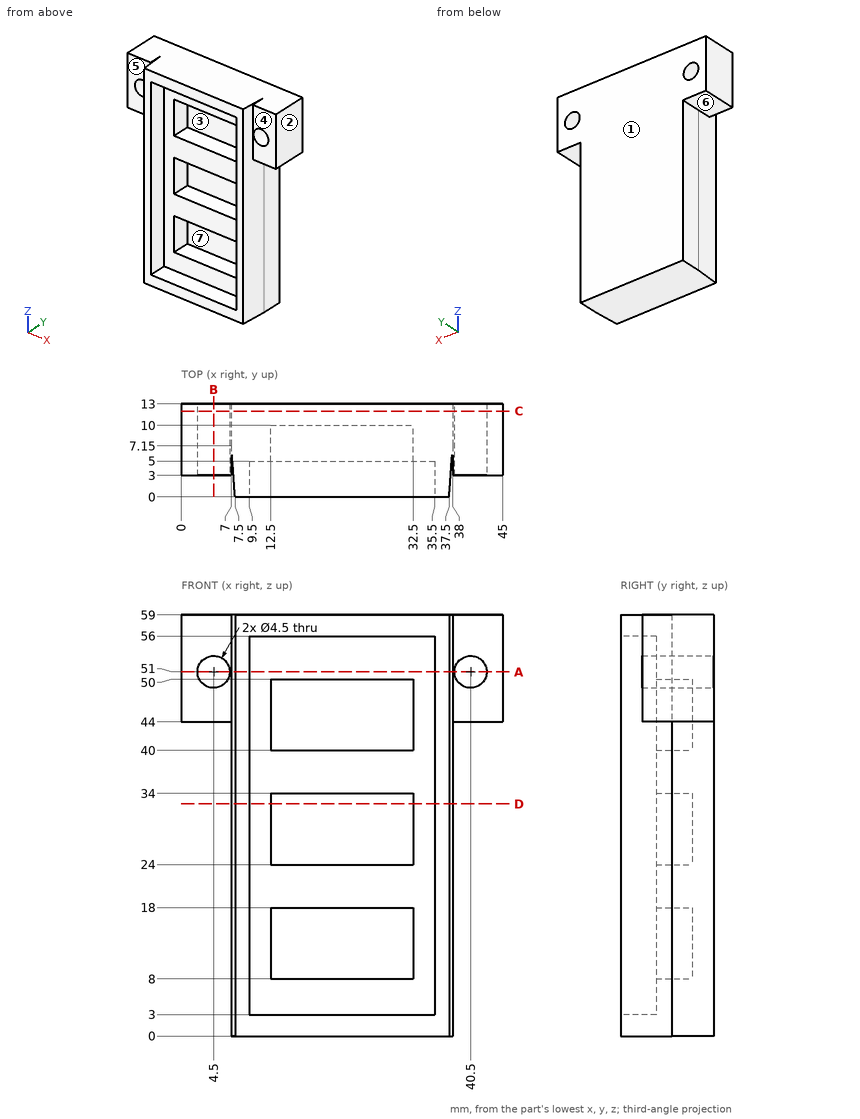
Print and shaded views of the part. All mm, measured from the part's lowest x, y and z. A direction names the side the tool comes from. Coordinates: 2 decimals unless noted, no trailing zeros. Loops run counter-clockwise (first coordinate to the right, second up) from the corner with the lowest first, then second, coordinate; pieces in that order, holes last. Notation, with made-up numbers: M 58.25,35.25 L 69.25,35.25 A12 cw 69.25,58.25 Z; hole C 86,33.5 d10. An arc over 180 degrees is marked long. Use a Markdown table: item, result. Add a question column.
Q1. Which spindle directions (+Z, -Z, +X, -X, +Y, -Y) get a long thin tool onto all of the face, cutting with end or side? Do the marked faces 4, 5, 6 and 7. Say none if no direction does.
Q2. Probe L1, parallel to Z at x = 18.5, y = 6; L2, parallel to X at y = 9.25, z = 51; L3, parallel to Z at x = 4.5, y = 10.75. List the from-to ranges inside material, lowest first.
Q3. Cut at B-B (x = 4.5). Write the cut outline in (y, z).
Q4. Mould opens along X. For the marked faces 1, 2 and 3 say: +X half, -X half, draft (parallel to the pull), parting line (faces both ways), or undercut.
Q5. Cut at D-D (z = 32.5). Write the cut outline in (x, y).
Q6. Cut at C-C (y = 12). Write the cut outline in (x, z), and give its area (3 significant figures).
Q7. Pin check, flat tips, straight feed: P1, Ø10, axis at x = 18.5, z = 25, coming from the -Y side; P2, Ø5, axis at x = 18.5, z = 28, coming from the -Y side; P3, Ø1.5, axis at y = 7.5, z = 12.5, coming from the +X side. Stop position of each tip, or through.
Q8. Cut at A-A (z = 51). Write the cut outline in (x, y).
Worked out:
| question | item | result |
|---|---|---|
| 1 | face 4 | +Z, -Z, +X, -Y |
| 1 | face 5 | +Z, -Z, -X, -Y |
| 1 | face 6 | -Z, -X, +Y, -Y |
| 1 | face 7 | -Y |
| 2 | L1 | z = 0 to 8, 18 to 24, 34 to 40, 50 to 59 |
| 2 | L2 | x = 0 to 2.25, 6.75 to 38.25, 42.75 to 45 |
| 2 | L3 | z = 44 to 48.75, 53.25 to 59 |
| 3 | outline | M 3,44 L 13,44 L 13,48.75 L 3,48.75 Z; M 3,53.25 L 13,53.25 L 13,59 L 3,59 Z |
| 4 | face 1 | draft |
| 4 | face 2 | +X half |
| 4 | face 3 | undercut |
| 5 | outline | M 7,7.15 L 7.5,0 L 9.5,0 L 9.5,5 L 12.5,5 L 12.5,10 L 32.5,10 L 32.5,5 L 35.5,5 L 35.5,0 L 37.5,0 L 38,7.15 L 38,13 L 7,13 Z |
| 6 | outline | M 0,44 L 7,44 L 7,0 L 38,0 L 38,44 L 45,44 L 45,59 L 0,59 Z; hole C 4.5,51 d4.5; hole C 40.5,51 d4.5 |
| 6 | area | 2,010 mm2 |
| 7 | P1 | stops at y = 5 |
| 7 | P2 | stops at y = 10 |
| 7 | P3 | stops at x = 38 |
| 8 | outline | M 0,3 L 2.25,3 L 2.25,13 L 0,13 Z; M 6.75,3 L 7,3 L 7,7.15 L 7.5,0 L 9.5,0 L 9.5,5 L 35.5,5 L 35.5,0 L 37.5,0 L 38,7.15 L 38,3 L 38.25,3 L 38.25,13 L 6.75,13 Z; M 42.75,3 L 45,3 L 45,13 L 42.75,13 Z |
